Geometry check sheet. Reference: drawing and pictorial views, mm from the part's lowest x, y, z. Round coordinates to 2 decimals unless told otherwise and drop trailing zeros. Order: outer loops, then holes, each group sorted by start corner. A loop starts at its lowest first (then second) coordinate and runs counter-clockwise, first axis right, second up.
Q1. Depth check by flat-ended pin: P1, Ø1, axis at y = 13, z = 3.5, coming from the -X side; P2, Ø1, axis at x = 4.5, y = 12, coming from the -Z side. Enter the tip coordinate at first touch or a pass-through.
Q2. Mould release check, pull along Z, two halves, no side actions. Record for the marked faces 1, 2 and 3: +Z half, -Z half, draft (parallel to the pull), parting line (faces both ways), or undercut.
Q3. Cross-section at C-C on x = 3. Record the cut outline in (y, z) (1 decimal).
Q4. Cross-section at A-A on y = 37.5. Record the cut outline in (x, z) (1 decimal), then the cut area to 3 significant figures.
Q5. Cross-section at D-D on z = 0.5. Record the cut outline in (x, y).
Q6. Cross-section at B-B on z = 2.45. Record the cut outline in (x, y) (1 decimal).
Q7. Scan lines: probe 1 along Z at (x, y) = (1.85, 10) (1 decimal); probe 2 along X at (y, z) = (31.5, 3.3) (1 decimal); probe 3 along X at (y, z) = (9, 2.1) (1 decimal). Record each from-to range of solid material in increasing order.
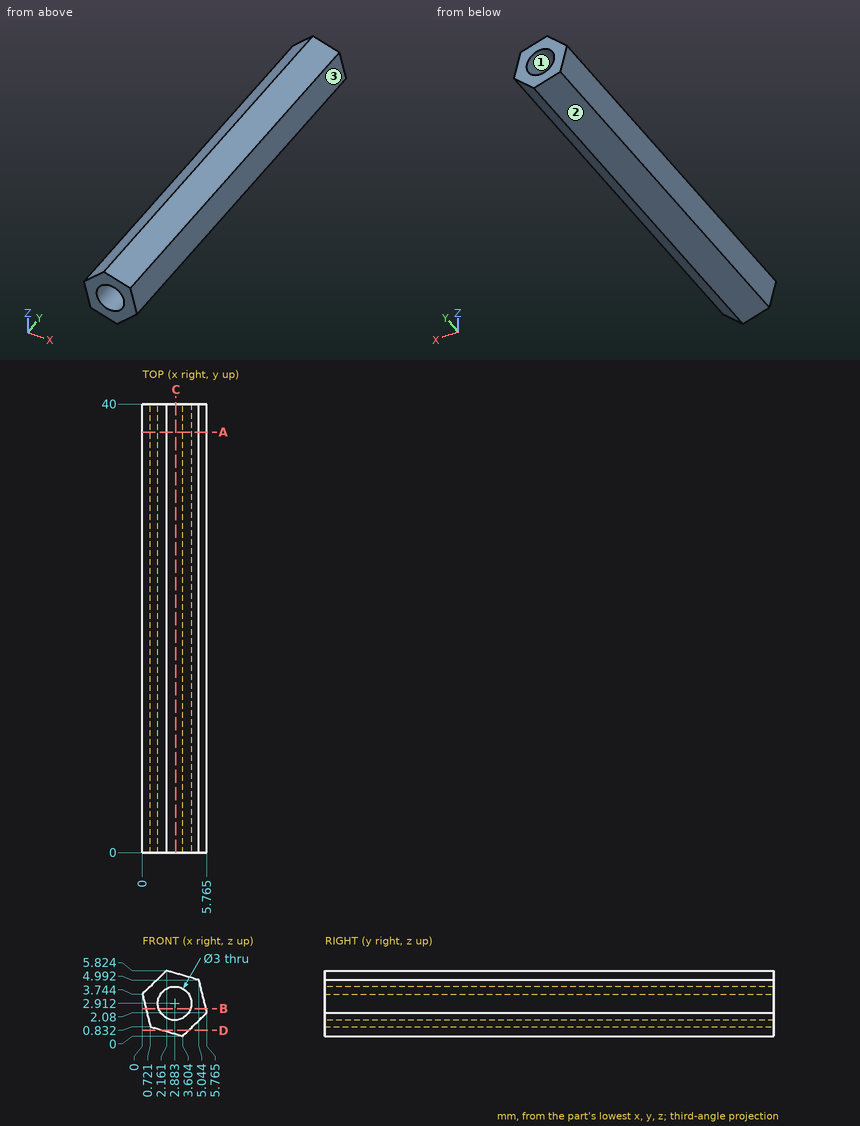
Results found:
1. P1: stops at x = 0
1. P2: stops at z = 0.38
2. face 1: undercut
2. face 2: -Z half
2. face 3: +Z half
3. outline: (0, 0.2) - (40, 0.2) - (40, 1.4) - (0, 1.4) - close; (0, 4.4) - (40, 4.4) - (40, 5.6) - (0, 5.6) - close
4. outline: (0, 3.7) - (0.7, 0.8) - (3.6, 0) - (5.8, 2.1) - (5, 5) - (2.2, 5.8) - close; hole circle Ø3 at (2.9, 2.9)
4. area: 16.3 mm2
5. outline: (1.87, 0) - (4.12, 0) - (4.12, 40) - (1.87, 40) - close
6. outline: (0.3, 0) - (1.5, 0) - (1.5, 40) - (0.3, 40) - close; (4.3, 0) - (5.7, 0) - (5.7, 40) - (4.3, 40) - close
7. probe 1: z = 0.5 to 1.8, 4 to 5.5
7. probe 2: x = 0.1 to 1.4, 4.3 to 5.5
7. probe 3: x = 0.4 to 1.6, 4.1 to 5.8
